from build123d import *

# Parameters (mm, degrees)
SKETCH1_W                                           = 150
SKETCH1_H                                           = 55
BOSS_EXTRUDE1_DEPTH                                 = 10
CSK_FOR_M4_COUNTERSUNK_FLAT_HEAD_SCREW1_D           = 4.5
CSK_FOR_M4_COUNTERSUNK_FLAT_HEAD_SCREW1_CSINK_D     = 9.4
CSK_FOR_M4_COUNTERSUNK_FLAT_HEAD_SCREW1_CSINK_ANGLE = 90
SKETCH4_W                                           = 100
SKETCH4_H                                           = 60
BOSS_EXTRUDE2_DEPTH                                 = 6
SKETCH5_W                                           = 99.587167191
SKETCH5_H                                           = 40.554359572
BOSS_EXTRUDE3_DEPTH                                 = 10
SKETCH6_R                                           = 6.325350673
BOSS_EXTRUDE4_DEPTH                                 = 10
SKETCH7_R                                           = 6.761038659
SKETCH7_W                                           = 5.613398263
SKETCH7_H                                           = 5.940244602
BOSS_EXTRUDE5_DEPTH                                 = 5
SKETCH8_R                                           = 7.825257062
BOSS_EXTRUDE6_DEPTH                                 = 20


with BuildPart() as part:
    # Sketch1 → Boss-Extrude1 (new body)
    with BuildSketch(Plane.XY):
        Rectangle(SKETCH1_W, SKETCH1_H)
    extrude(amount=BOSS_EXTRUDE1_DEPTH)

    # CSK for M4 Countersunk Flat Head Screw1 (through all)
    with Locations(Plane(origin=(0, 0, 0), x_dir=(-1, 0, 0), z_dir=(0, 0, -1))):
        with Locations((-72, 24), (-72, -24.31977753), (72, -24), (72, 24)):
            CounterSinkHole(CSK_FOR_M4_COUNTERSUNK_FLAT_HEAD_SCREW1_D / 2, CSK_FOR_M4_COUNTERSUNK_FLAT_HEAD_SCREW1_CSINK_D / 2, counter_sink_angle=CSK_FOR_M4_COUNTERSUNK_FLAT_HEAD_SCREW1_CSINK_ANGLE)

    # Sketch4 → Boss-Extrude2 (add)
    with BuildSketch(Plane(origin=(0, 0, 0), x_dir=(-1, 0, 0), z_dir=(0, 0, -1))):
        with Locations((-12.709987385, -7.767861044)):
            Rectangle(SKETCH4_W, SKETCH4_H)
    extrude(amount=BOSS_EXTRUDE2_DEPTH)

    # Sketch5 → Boss-Extrude3 (add)
    with BuildSketch(Plane(origin=(0, 0, -6), x_dir=(-1, 0, 0), z_dir=(0, 0, -1))):
        with Locations((-12.91640379, -7.112004415)):
            Rectangle(SKETCH5_W, SKETCH5_H)
    extrude(amount=BOSS_EXTRUDE3_DEPTH)

    # Sketch6 → Boss-Extrude4 (add)
    with BuildSketch(Plane(origin=(0, 0, 0), x_dir=(-1, 0, 0), z_dir=(0, 0, -1))):
        with Locations(Location((59.771620242, 16.04141059, 0), (0, 0, 180))):
            Circle(SKETCH6_R)
    extrude(amount=BOSS_EXTRUDE4_DEPTH)

    # Sketch7 → Boss-Extrude5 (add)
    with BuildSketch(Plane(origin=(0, 0, 0), x_dir=(-1, 0, 0), z_dir=(0, 0, -1))):
        with Locations(Location((60.574566505, -3.736064786, 0), (0, 0, 180))):
            Circle(SKETCH7_R)
        with Locations((60.574566506, -19.28347932)):
            Rectangle(SKETCH7_W, SKETCH7_H)
    extrude(amount=BOSS_EXTRUDE5_DEPTH)

    # Sketch8 → Boss-Extrude6 (add)
    with BuildSketch(Plane(origin=(0, 0, -5), x_dir=(-1, 0, 0), z_dir=(0, 0, -1))):
        with Locations((60.574566505, -3.736064786)):
            Circle(SKETCH8_R)
    extrude(amount=BOSS_EXTRUDE6_DEPTH)


solid = part.part
Geometry: final body of the model. Coordinates: model frame, mm. A direction names the side the tool comes from. Give positions to 0.01 mm unless a question says otherwise; leave off trailing zeros. Loops run counter-clockwise (first coordinate to the right, second up) from the corner with the lowest first, then second, coordinate; pieces in that order, holes last. Notation, with made-up numbers: (76, 33.25) -> (134, 33.25) arc R25 cw to (134, 54.25) -> close; hole circle Ø4 at (29.25, 78). An arc over 180 degrees is marked (long way). Put each result on its own line as item: value.
1. Pull-direction query (Y, two-part tool) for faces 1 (the flat face through (-1, 27.5, 5)), 2 (the flat face through (9, -28, -6)), 3 (the cylindrical face through (-70.962, -25.996, 6.278)); classes: released by +Y, released by -Y, zero draft, split by the parting line, or undercut.
Taken from the geometry:
face 1: released by +Y
face 2: zero draft
face 3: undercut
2. Ray query, line 1 along Y through (x, z) = (72, 5); line 2 along Y through (x, z) = (-72, 7.5); line 3 along X through (y, z) = (24, 6.5). Return the intervals inside material, ascending. Write a range as [from, to].
Taken from the geometry:
line 1: y = [-27.5, -26.57], [-22.07, 21.75], [26.25, 27.5]
line 2: y = [-27.5, -26.25], [-21.75, 21.75], [26.25, 27.5]
line 3: x = [-75, -74.25], [-69.75, 69.75], [74.25, 75]
3. Pin query (flat end, axial travel): P1, Ø3, axis at x = 58.5, y = -31, coming from the +Z side; P2, Ø3, axis at y = -22.5, z = -4, coming from the -X side; P3, Ø11, axis at y = -5.5, z = -9, coming from the -X side; P4, Ø2.5, axis at x = -72, y = -24, coming from the +Z side. Return the tip coordinate at first contact, or that it passes through.
Taken from the geometry:
P1: stops at z = 0
P2: stops at x = -63.38
P3: stops at x = -68.4
P4: passes through
4. Cut plane C-C (z = 4.5). Return the cut outline in (x, y), plus the area to 3 significant figures.
Taken from the geometry:
outline: (-75, -27.5) -> (75, -27.5) -> (75, 27.5) -> (-75, 27.5) -> close; hole circle Ø4.5 at (-72, -24); hole circle Ø4.5 at (-72, 24); hole circle Ø4.5 at (72, -24.32); hole circle Ø4.5 at (72, 24)
area: 8,190 mm2
5. Cut plane A-A (y = 24). Return the cut outline in (x, z), plus the area to 3 significant figures.
Taken from the geometry:
outline: (-75, 1.7) -> (-74.25, 2.45) -> (-74.25, 10) -> (-75, 10) -> close; (-69.75, 2.45) -> (-67.3, 0) -> (67.3, 0) -> (69.75, 2.45) -> (69.75, 10) -> (-69.75, 10) -> close; (74.25, 2.45) -> (75, 1.7) -> (75, 10) -> (74.25, 10) -> close
area: 1,400 mm2
6. Cut plane D-D (x = 13). Return the cut outline in (y, z).
Taken from the geometry:
outline: (-37.77, -6) -> (-27.39, -6) -> (-27.39, -16) -> (13.17, -16) -> (13.17, -6) -> (22.23, -6) -> (22.23, 0) -> (27.5, 0) -> (27.5, 10) -> (-27.5, 10) -> (-27.5, 0) -> (-37.77, 0) -> close
7. Set-up query: faces 4 (the cylindrical face through (-64.434, 11.766, -4.93)), 5 (the flat face through (-54, -6, -5)), 6 (the flat face through (-61, -22.254, -2)), 7 (the flat face through (-1, -27.5, 5)). Return all of +Z, -Z, +X, -X, +Y, -Y with unobstructed straight access to the full face (end or side cutting, diameter ignored); none if empty.
Taken from the geometry:
face 4: -Z
face 5: none
face 6: -Z, -X, -Y
face 7: +Z, +X, -X, -Y
8. Cut plane B-B (x = -72). Return the cut outline in (y, z).
Taken from the geometry:
outline: (-27.5, 1.2) -> (-26.25, 2.45) -> (-26.25, 10) -> (-27.5, 10) -> close; (-21.75, 2.45) -> (-19.3, 0) -> (19.3, 0) -> (21.75, 2.45) -> (21.75, 10) -> (-21.75, 10) -> close; (26.25, 2.45) -> (27.5, 1.2) -> (27.5, 10) -> (26.25, 10) -> close
